Work out the finished part from the listing and answer in its coordinate system (mm). A direction names the side the tool comes from. Round coordinates to 2 decimals unless told otherwise and drop trailing zeros. Loops run counter-clockwise (first coordinate to the right, second up) from the corner with the lowest first, then second, coordinate; pieces in that order, holes last. Notation, with made-up numbers: (31.5, 61) -> (76.5, 61) arc R35 cw to (76.5, 100) -> close; hole circle Ø5 at (26, 29.5). An arc over 180 degrees is marked (long way). Use one line per item in the form item = value.
```python
from build123d import *

# Parameters (mm, degrees)
SKETCH1_W            = 19.82
SKETCH1_H            = 39.88
BOSS_EXTRUDE1_DEPTH  = 36.02
SKETCH2_W            = 19.82
SKETCH2_H            = 6.6
BOSS_EXTRUDE2_DEPTH  = 2.54
CUT_EXTRUDE1_DEPTH   = 2.54
SKETCH4_W            = 1
SKETCH4_H            = 6.6
BOSS_EXTRUDE3_DEPTH  = 1.5
CUT_EXTRUDE2_DEPTH   = 1
SKETCH6_W            = 19.82
SKETCH6_H            = 39.88
CUT_EXTRUDE3_DEPTH   = 3.55
SKETCH7_W            = 18.22
SKETCH7_H            = 38.272033082
BOSS_EXTRUDE4_DEPTH  = 0.762
FILLET1_R            = 1.27
FILLET2_R            = 0.762
BOSS_EXTRUDE5_DEPTH  = 2.54
SKETCH10_R           = 6.477
BOSS_EXTRUDE6_DEPTH  = 2.286
SKETCH11_R           = 5.461
BOSS_EXTRUDE7_DEPTH  = 0.762
SKETCH12_R           = 1.75
CUT_EXTRUDE4_DEPTH   = 2.54
SKETCH13_W           = 17.371497452
SKETCH13_H           = 10
SKETCH13_W_2         = 15.847497452
SKETCH13_H_2         = 8.476
BOSS_EXTRUDE8_DEPTH  = 0.254
BOSS_EXTRUDE9_DEPTH  = 2.54
CUT_EXTRUDE5_DEPTH   = 1.524
SKETCH16_R           = 0.5
CUT_EXTRUDE6_DEPTH   = 6
CHAMFER1_SIZE        = 1
FILLET3_R            = 0.5
SKETCH17_W           = 6.35
SKETCH17_H           = 3.81
BOSS_EXTRUDE10_DEPTH = 1.5
FILLET5_R            = 0.5
FILLET6_R            = 1


with BuildPart() as part:
    # Sketch1 → Boss-Extrude1 (new body)
    with BuildSketch(Plane(origin=(0, 0, 0), x_dir=(1, 0, 0), z_dir=(0, 1, 0))):
        Rectangle(SKETCH1_W, SKETCH1_H)
    extrude(amount=BOSS_EXTRUDE1_DEPTH)

    # Sketch2 → Boss-Extrude2 (add)
    with BuildSketch(Plane(origin=(0, 26.67, 0), x_dir=(1, 0, 0), z_dir=(0, 1, 0))):
        with Locations((0, 23.24)):
            Rectangle(SKETCH2_W, SKETCH2_H)
        with Locations((0, -23.24)):
            Rectangle(SKETCH2_W, SKETCH2_H)
    extrude(amount=BOSS_EXTRUDE2_DEPTH)

    # Sketch3 → Cut-Extrude1 (cut)
    with BuildSketch(Plane(origin=(0, 29.21, 0), x_dir=(1, 0, 0), z_dir=(0, 1, 0))):
        with BuildLine():
            Line((6.355, 26.54), (3.555, 26.54))
            Line((3.555, 26.54), (3.555, 25.539072445))
            ThreePointArc((3.555, 25.539072445), (4.955, 21.665), (6.355, 25.539072445))
            Line((6.355, 25.539072445), (6.355, 26.54))
        make_face()
        with BuildLine():
            Line((-6.355, 26.54), (-6.355, 25.539072445))
            ThreePointArc((-6.355, 25.539072445), (-4.955, 21.665), (-3.555, 25.539072445))
            Line((-3.555, 25.539072445), (-3.555, 26.54))
            Line((-3.555, 26.54), (-6.355, 26.54))
        make_face()
    cut_extrude1 = extrude(amount=-CUT_EXTRUDE1_DEPTH, mode=Mode.SUBTRACT)

    # Mirror1: Cut-Extrude1 across plane
    add(cut_extrude1.mirror(Plane.XY), mode=Mode.SUBTRACT)

    # Sketch4 → Boss-Extrude3 (add)
    with BuildSketch(Plane(origin=(0, 29.21, 0), x_dir=(1, 0, 0), z_dir=(0, 1, 0))):
        with Locations((0, 23.24)):
            Rectangle(SKETCH4_W, SKETCH4_H)
        with Locations((0, -23.24)):
            Rectangle(SKETCH4_W, SKETCH4_H)
    extrude(amount=BOSS_EXTRUDE3_DEPTH)

    # Sketch5 → Cut-Extrude2 (cut)
    with BuildSketch(Plane.ZY.offset(0.5)):
        Polygon((-26.54, 29.21), (-25.54, 30.71), (-26.54, 30.71), align=None)
        Polygon((26.54, 30.71), (26.54, 29.21), (25.54, 30.71), align=None)
    extrude(amount=-CUT_EXTRUDE2_DEPTH, mode=Mode.SUBTRACT)

    # Sketch6 → Cut-Extrude3 (cut)
    with BuildSketch(Plane(origin=(0, 36.02, 0), x_dir=(1, 0, 0), z_dir=(0, 1, 0))):
        Rectangle(SKETCH6_W, SKETCH6_H)
    extrude(amount=-CUT_EXTRUDE3_DEPTH, mode=Mode.SUBTRACT)

    # Sketch7 → Boss-Extrude4 (add)
    with BuildSketch(Plane(origin=(0, 32.47, 0), x_dir=(1, 0, 0), z_dir=(0, 1, 0))):
        Rectangle(SKETCH7_W, SKETCH7_H)
    extrude(amount=BOSS_EXTRUDE4_DEPTH)

    # Fillet1
    fillet1_edges = [part.edges().sort_by_distance(p)[0] for p in [
        (-9.91, 13.335, -19.94),
        (-9.91, 30.84, -19.94),
        (9.91, 13.335, -19.94),
        (9.91, 30.84, -19.94),
        (9.91, 13.335, 19.94),
        (9.91, 30.84, 19.94),
        (-9.91, 13.335, 19.94),
        (-9.91, 30.84, 19.94),
    ]]
    fillet(fillet1_edges, radius=FILLET1_R)

    # Fillet2
    fillet2_edges = [part.edges().sort_by_distance(p)[0] for p in [
        (9.11, 32.851, -19.136016541),
        (-9.11, 32.851, -19.136016541),
        (-9.11, 32.851, 19.136016541),
        (9.11, 32.851, 19.136016541),
    ]]
    fillet(fillet2_edges, radius=FILLET2_R)

    # Sketch8 → Boss-Extrude5 (add)
    with BuildSketch(Plane(origin=(0, 33.232, 0), x_dir=(1, 0, 0), z_dir=(0, 1, 0))):
        with BuildLine():
            Line((8.685748726, 7.213983459), (8.685748726, -12.786016541))
            Line((8.685748726, -12.786016541), (-8.685748726, -12.786016541))
            Line((-8.685748726, -12.786016541), (-8.685748726, 7.213983459))
            ThreePointArc((-8.685748726, 7.213983459), (0, 19.136016541), (8.685748726, 7.213983459))
        make_face()
    extrude(amount=BOSS_EXTRUDE5_DEPTH)

    # Sketch10 → Boss-Extrude6 (add)
    with BuildSketch(Plane(origin=(0, 35.772, 0), x_dir=(1, 0, 0), z_dir=(0, 1, 0))):
        with Locations(Location((0, 10.011016541, 0), (0, 0, 270))):
            Circle(SKETCH10_R)
    extrude(amount=BOSS_EXTRUDE6_DEPTH)

    # Sketch11 → Boss-Extrude7 (add)
    with BuildSketch(Plane(origin=(0, 38.058, 0), x_dir=(1, 0, 0), z_dir=(0, 1, 0))):
        with Locations(Location((0, 10.011016541, 0), (0, 0, 90))):
            Circle(SKETCH11_R)
    extrude(amount=BOSS_EXTRUDE7_DEPTH)

    # Sketch12 → Cut-Extrude4 (cut)
    with BuildSketch(Plane(origin=(0, 38.82, 0), x_dir=(1, 0, 0), z_dir=(0, 1, 0))):
        with Locations(Location((0, 10.011016541, 0), (0, 0, 270))):
            Circle(SKETCH12_R)
    extrude(amount=-CUT_EXTRUDE4_DEPTH, mode=Mode.SUBTRACT)

    # Sketch13 → Boss-Extrude8 (add)
    with BuildSketch(Plane(origin=(0, 35.772, 0), x_dir=(1, 0, 0), z_dir=(0, 1, 0))):
        with Locations((0, -7.786016541)):
            Rectangle(SKETCH13_W, SKETCH13_H)
        with Locations((0, -7.786016541)):
            Rectangle(SKETCH13_W_2, SKETCH13_H_2, mode=Mode.SUBTRACT)
    extrude(amount=BOSS_EXTRUDE8_DEPTH)

    # Sketch14 → Boss-Extrude9 (add)
    with BuildSketch(Plane(origin=(0, 33.232, 0), x_dir=(1, 0, 0), z_dir=(0, 1, 0))):
        with BuildLine():
            Line((-4.260362688, -12.786016541), (4.260362688, -12.786016541))
            ThreePointArc((4.260362688, -12.786016541), (0, -14.354935039), (-4.260362688, -12.786016541))
        make_face()
    extrude(amount=BOSS_EXTRUDE9_DEPTH)

    # Sketch15 → Cut-Extrude5 (cut)
    with BuildSketch(Plane(origin=(0, 0, 0), x_dir=(-1, 0, 0), z_dir=(0, -1, 0))):
        with BuildLine():
            Line((6.46365167, -19.94), (9.91, -19.94))
            Line((9.91, -19.94), (9.91, -16.211847956))
            ThreePointArc((9.91, -16.211847956), (7.678426739, -17.605953774), (6.46365167, -19.94))
        make_face()
        with BuildLine():
            Line((-9.91, -19.94), (-9.91, -16.211847956))
            ThreePointArc((-9.91, -16.211847956), (-7.678426739, -17.605953774), (-6.46365167, -19.94))
            Line((-6.46365167, -19.94), (-9.91, -19.94))
        make_face()
        with BuildLine():
            Line((-6.46365167, 19.94), (-9.91, 19.94))
            Line((-9.91, 19.94), (-9.91, 16.211847956))
            ThreePointArc((-9.91, 16.211847956), (-7.678426739, 17.605953774), (-6.46365167, 19.94))
        make_face()
        with BuildLine():
            Line((9.91, 19.94), (9.91, 16.211847956))
            ThreePointArc((9.91, 16.211847956), (7.678426739, 17.605953774), (6.46365167, 19.94))
            Line((6.46365167, 19.94), (9.91, 19.94))
        make_face()
    extrude(amount=-CUT_EXTRUDE5_DEPTH, mode=Mode.SUBTRACT)

    # Sketch16 → Cut-Extrude6 (cut)
    with BuildSketch(Plane(origin=(0, 0, 0), x_dir=(-1, 0, 0), z_dir=(0, -1, 0))):
        with Locations(Location((8.64, -18.67, 0), (0, 0, 90))):
            Circle(SKETCH16_R)
        with Locations(Location((-8.64, -18.67, 0), (0, 0, 270))):
            Circle(SKETCH16_R)
        with Locations(Location((-8.64, 18.67, 0), (0, 0, 90))):
            Circle(SKETCH16_R)
        with Locations(Location((8.64, 18.67, 0), (0, 0, 270))):
            Circle(SKETCH16_R)
    extrude(amount=-CUT_EXTRUDE6_DEPTH, mode=Mode.SUBTRACT)

    # Chamfer1
    chamfer1_edges = [part.edges().sort_by_distance(p)[0] for p in [
        (0, 0, 19.94),
        (9.91, 0, 0),
        (0, 0, -19.94),
        (-9.91, 0, 0),
    ]]
    chamfer(chamfer1_edges, length=CHAMFER1_SIZE)

    # Fillet3
    fillet3_edges = [part.edges().sort_by_distance(p)[0] for p in [
        (-7.678426739, 1.524, 17.605953774),
        (7.678426739, 1.524, 17.605953774),
        (7.678426739, 1.524, -17.605953774),
        (-7.678426739, 1.524, -17.605953774),
    ]]
    fillet(fillet3_edges, radius=FILLET3_R)

    # Sketch17 → Boss-Extrude10 (add)
    with BuildSketch(Plane(origin=(0, 0, -19.94), x_dir=(-1, 0, 0), z_dir=(0, 0, -1))):
        with Locations((0, 2.905)):
            Rectangle(SKETCH17_W, SKETCH17_H)
        Polygon((0, 1.5), (-2.675, 1.5), (-2.675, 4.31), (0, 4.31), (2.675, 4.31), (2.675, 1.5), align=None, mode=Mode.SUBTRACT)
    extrude(amount=BOSS_EXTRUDE10_DEPTH)

    # Fillet5
    fillet5_edges = [part.edges().sort_by_distance(p)[0] for p in [
        (3.175, 1, -20.69),
        (-3.175, 1, -20.69),
        (-3.175, 4.81, -20.69),
        (3.175, 4.81, -20.69),
    ]]
    fillet(fillet5_edges, radius=FILLET5_R)

    # Fillet6
    fillet6_edges = [part.edges().sort_by_distance(p)[0] for p in [
        (9.91, 27.94, 26.54),
        (9.91, 27.94, -26.54),
        (-9.91, 27.94, 26.54),
        (-9.91, 27.94, -26.54),
    ]]
    fillet(fillet6_edges, radius=FILLET6_R)


solid = part.part
```
(1) Find section A-A, the plane z = -2. Write down the section's boundary in (x, y), then the cut area to 3 significant figures.
Completed:
outline = (-9.91, 1) -> (-8.91, 0) -> (8.91, 0) -> (9.91, 1) -> (9.91, 32.47) -> (9.11, 32.47) -> (9.11, 33.23) -> (8.69, 33.23) -> (8.69, 35.77) -> (-8.69, 35.77) -> (-8.69, 33.23) -> (-9.11, 33.23) -> (-9.11, 32.47) -> (-9.91, 32.47) -> close
area = 701 mm2
(2) Find section B-B, the plane y = 11.5. Write down the section's boundary in (x, z).
Completed:
outline = (-9.91, -18.67) arc R1.27 ccw to (-8.64, -19.94) -> (8.64, -19.94) arc R1.27 ccw to (9.91, -18.67) -> (9.91, 18.67) arc R1.27 ccw to (8.64, 19.94) -> (-8.64, 19.94) arc R1.27 ccw to (-9.91, 18.67) -> close
(3) Find section C-C, the plane z = 20.5. Write down the section's boundary in (x, y), then the cut area to 3 significant figures.
Completed:
outline = (-9.91, 26.67) -> (9.91, 26.67) -> (9.91, 29.21) -> (0.5, 29.21) -> (0.5, 30.71) -> (-0.5, 30.71) -> (-0.5, 29.21) -> (-9.91, 29.21) -> close
area = 51.8 mm2
(4) For a pull along Y with two mould halves and no side action, classify faces 1 (the flat face through (0, 4.31, -21)), 2 (the cylindrical face through (-5.03, 27.958, 21.666)), 3 (the flat face through (-6.3, 29.21, -21.8)), 4 (the flat face through (0, 26.67, 23)) as +Y half, -Y half, draft (parallel to the pull), parting line (faces both ways), or undercut.
Completed:
face_1 = undercut
face_2 = draft
face_3 = +Y half
face_4 = -Y half
(5) Given P1, Ø5, axis at x = -1.5, y = 19, coming from the +Z side; P2, Ø0.9, axis at x = 8.5, z = 18, coming from the -Y side; P3, Ø8, axis at x = 1, y = 11.5, coming from the -Z side, each flat-ended and moving along its own axis, determine where each tip first touches the part or whether it passes through.
Completed:
P1 = 19.94
P2 = 1.52
P3 = -19.94
(6) For faces 5 (the cylindrical face through (-9.548, 30.863, -19.558)), 6 (the cylindrical face through (1.183, 37.568, -11.301)), 7 (the cylindrical face through (-9.548, 14.273, 19.558)), 8 (the flat face through (0, 4.81, -21)), determine the directions among +Z, -Z, +X, -X, +Y, -Y from which every point of the face is accessible in a straight line to the end or side of a thin tool.
Completed:
face_5 = -Z, -X, +Y
face_6 = +Y
face_7 = +Z, -X, -Y
face_8 = -Z, +X, -X
(7) Consider L1, parallel to X at y = 3.95, z = 18.67; L2, parallel to Z at x = 3.25, y = 28; L3, parallel to Y at x = -2, z = -0.5. Determine where each line is inside the solid, lowest interval first.
Completed:
L1 = -9.91 to -9.14, -8.14 to 8.14, 9.14 to 9.91
L2 = -26.54 to -25.23, -22.48 to 22.48, 25.23 to 26.54
L3 = 0 to 35.77
